from build123d import *

# Parameters (mm, degrees)
SKETCH084_W     = 81.6
SKETCH084_H     = 39.6
PAD023_DEPTH    = 34.3
FILLET002_R     = 3
POCKET007_DEPTH = 1.2
POCKET019_DEPTH = 1.2
POCKET016_DEPTH = 1.2
POCKET021_DEPTH = 1.2
POCKET020_DEPTH = 1.2
POCKET018_DEPTH = 1.2
SKETCH094_R     = 6.6
SKETCH094_R_2   = 9.4
SKETCH094_R_3   = 5.3
POCKET017_DEPTH = 34.301


with BuildPart() as part:
    # Sketch084 → Pad023 (new body)
    with BuildSketch(Plane.XY):
        with Locations((42, 21)):
            Rectangle(SKETCH084_W, SKETCH084_H)
    extrude(amount=PAD023_DEPTH)

    # Fillet002
    fillet002_edges = [part.edges().sort_by_distance(p)[0] for p in [
        (82.8, 1.2, 17.15),
        (1.2, 1.2, 17.15),
        (1.2, 40.8, 17.15),
        (82.8, 40.8, 17.15),
    ]]
    fillet(fillet002_edges, radius=FILLET002_R)

    # Sketch088 → Pocket007 (cut)
    with BuildSketch(Plane(origin=(2, 7, 0), x_dir=(1, 0, 0), z_dir=(0, -1, 0))):
        with BuildLine():
            ThreePointArc((1.5, 25.5), (27, 0), (52.5, 25.5))
            Line((52.5, 61.679322), (52.5, 25.5))
            Line((1.5, 61.679322), (52.5, 61.679322))
            Line((1.5, 25.5), (1.5, 61.679322))
        make_face()
    extrude(amount=-POCKET007_DEPTH, mode=Mode.SUBTRACT)

    # Sketch089 → Pocket019 (cut)
    with BuildSketch(Plane(origin=(2, 13, 0), x_dir=(1, 0, 0), z_dir=(0, -1, 0))):
        with BuildLine():
            ThreePointArc((4.5, 28.5), (26.999982, 6), (49.5, 28.499964))
            Line((49.5, 51.5), (49.5, 28.499964))
            Line((4.5, 51.5), (49.5, 51.5))
            Line((4.5, 28.5), (4.5, 51.5))
        make_face()
    extrude(amount=-POCKET019_DEPTH, mode=Mode.SUBTRACT)

    # Sketch090 → Pocket016 (cut)
    with BuildSketch(Plane(origin=(2, 18, 0), x_dir=(1, 0, 0), z_dir=(0, -1, 0))):
        with BuildLine():
            ThreePointArc((9.3, 33.3), (26.999984, 15.6), (44.7, 33.299969))
            Line((44.7, 56.3), (44.7, 33.299969))
            Line((9.3, 56.3), (44.7, 56.3))
            Line((9.3, 33.3), (9.3, 56.3))
        make_face()
    extrude(amount=-POCKET016_DEPTH, mode=Mode.SUBTRACT)

    # Sketch091 → Pocket021 (cut)
    with BuildSketch(Plane(origin=(2, 23, 0), x_dir=(1, 0, 0), z_dir=(0, -1, 0))):
        with BuildLine():
            ThreePointArc((10.8, 34.8), (26.999981, 18.6), (43.2, 34.799961))
            Line((43.2, 57.8), (43.2, 34.799961))
            Line((10.8, 57.8), (43.2, 57.8))
            Line((10.8, 34.8), (10.8, 57.8))
        make_face()
    extrude(amount=-POCKET021_DEPTH, mode=Mode.SUBTRACT)

    # Sketch092 → Pocket020 (cut)
    with BuildSketch(Plane(origin=(2, 28, 0), x_dir=(1, 0, 0), z_dir=(0, -1, 0))):
        with BuildLine():
            ThreePointArc((14.4, 38.4), (26.999981, 25.8), (39.6, 38.399963))
            Line((39.6, 61.4), (39.6, 38.399963))
            Line((14.4, 61.4), (39.6, 61.4))
            Line((14.4, 38.4), (14.4, 61.4))
        make_face()
    extrude(amount=-POCKET020_DEPTH, mode=Mode.SUBTRACT)

    # Sketch093 → Pocket018 (cut)
    with BuildSketch(Plane(origin=(2, 34, 0), x_dir=(1, 0, 0), z_dir=(0, -1, 0))):
        with BuildLine():
            ThreePointArc((15.8, 39.8), (26.999979, 28.6), (38.2, 39.799958))
            Line((38.2, 62.8), (38.2, 39.799958))
            Line((15.8, 62.8), (38.2, 62.8))
            Line((15.8, 39.8), (15.8, 62.8))
        make_face()
    extrude(amount=-POCKET018_DEPTH, mode=Mode.SUBTRACT)

    # Sketch094 → Pocket017 (cut, through all)
    with BuildSketch(Plane.XY):
        with Locations((75, 32.3)):
            Circle(SKETCH094_R)
        with Locations((75, 14.069301)):
            Circle(SKETCH094_R)
        with Locations((60.137726, 23.285616)):
            Circle(SKETCH094_R_2)
        with Locations((63.524133, 8.113385)):
            Circle(SKETCH094_R_3)
        with Locations((48.131386, 33.31328)):
            Circle(SKETCH094_R_3)
    extrude(amount=POCKET017_DEPTH, mode=Mode.SUBTRACT)


solid = part.part
Work out the finished part from the listing and answer in its coordinate system (mm). A direction names the side the tool comes from. Coordinates: 2 decimals unless noted, no trailing zeros. Loops run counter-clockwise (first coordinate to the right, second up) from the corner with the lowest first, then second, coordinate; pieces in that order, holes last. Notation, with made-up numbers: (-37.75, -19.5) -> (-29.75, -19.5) arc R11 cw to (-29.75, -8.5) -> close; hole circle Ø10 at (61.25, -40). An arc over 180 degrees is marked (long way). Write each question's results on one line, items separated by ' | '. Start each with the question number.
1) Find section B-B on y = 11.5. Determine the outline of the cut face in (x, z).
2) The mould has two halves that part along X. Classify faces 3 (the flat face through (1.2, 21, 17)), 4 (the flat face through (41, 40.8, 17)), 5 (the flat face through (29, 35.2, 32)): pulls with the +X half, pulls with the -X half, needs draft (parallel to the pull), parting line crosses it, or undercut.
3) For faces 1 (the cylindrical face through (58.23, 8.35, 16.91)), 2 (the flat face through (29, 23, 28)), determine the directions among +Z, -Z, +X, -X, +Y, -Y from which every point of the face is accessible in a straight line to the end or side of a thin tool.
4) Find section D-D on z = 12.5. Determine the outline of the cut face in (x, y), then the cut area to 3 significant figures.
5) Find section A-A on x = 75. Determine the outline of the cut face in (y, z).
6) Find section C-C on z = 27. Count the separate pieces of the cut face and the enclosed holes in it, then the cut area to 3 significant figures.
7) Consider line 1 along Y through (x, z) = (39.5, 32); line 2 along Y through (x, z) = (48, 15); line 3 along Y through (x, z) = (42, 25). Determine where each line is inside the solid, lowest interval first.
Response values:
1) outline: (1.2, 0) -> (59.45, 0) -> (59.45, 34.3) -> (1.2, 34.3) -> close; (67.6, 0) -> (68.92, 0) -> (68.92, 34.3) -> (67.6, 34.3) -> close; (81.08, 0) -> (82.8, 0) -> (82.8, 34.3) -> (81.08, 34.3) -> close
2) face 3: pulls with the -X half | face 4: needs draft | face 5: undercut
3) face 1: +Z, -Z | face 2: +Z
4) outline: (1.2, 4.2) arc R3 ccw to (4.2, 1.2) -> (79.8, 1.2) arc R3 ccw to (82.8, 4.2) -> (82.8, 37.8) arc R3 ccw to (79.8, 40.8) -> (4.2, 40.8) arc R3 ccw to (1.2, 37.8) -> close; hole (7.06, 7) -> (50.94, 7) -> (50.94, 8.2) -> (7.06, 8.2) -> close; hole (13.18, 13) -> (44.82, 13) -> (44.82, 14.2) -> (13.18, 14.2) -> close; hole circle Ø10.6 at (48.13, 33.31); hole circle Ø18.8 at (60.14, 23.29); hole circle Ø10.6 at (63.52, 8.11); hole circle Ø13.2 at (75, 14.07); hole circle Ø13.2 at (75, 32.3) | area: 2,410 mm^2
5) outline: (1.2, 0) -> (7.47, 0) -> (7.47, 34.3) -> (1.2, 34.3) -> close; (20.67, 0) -> (25.7, 0) -> (25.7, 34.3) -> (20.67, 34.3) -> close; (38.9, 0) -> (40.8, 0) -> (40.8, 34.3) -> (38.9, 34.3) -> close
6) separate pieces: 1 | enclosed holes: 10 | area: 2,290 mm^2
7) line 1: y = 1.2 to 7, 8.2 to 13, 14.2 to 18, 19.2 to 23, 24.2 to 28, 29.2 to 40.8 | line 2: y = 1.2 to 7, 8.2 to 28.01, 38.61 to 40.8 | line 3: y = 1.2 to 7, 8.2 to 13, 14.2 to 18, 19.2 to 40.8
